```python
from build123d import *

# Parameters (mm, degrees)
SKETCH2_R           = 125
BOSS_EXTRUDE1_DEPTH = 50
CUT_EXTRUDE1_START  = -30
CUT_EXTRUDE1_DEPTH  = 30


with BuildPart() as part:
    # Sketch2 → Boss-Extrude1 (new body)
    with BuildSketch(Plane(origin=(0, 0, 0), x_dir=(1, 0, 0), z_dir=(0, 1, 0))):
        with Locations(Location((0, 0, 0), (0, 0, 270))):
            Circle(SKETCH2_R)
    extrude(amount=BOSS_EXTRUDE1_DEPTH)

    # Sketch3 → Cut-Extrude1 (cut)
    with BuildSketch(Plane(origin=(0, 50, 0), x_dir=(1, 0, 0), z_dir=(0, 1, 0)).offset(CUT_EXTRUDE1_START)):
        with BuildLine():
            Line((-122.662612071, 24.06), (122.662612071, 24.06))
            ThreePointArc((122.662612071, 24.06), (111.692828355, 56.122295874), (92.51441185, 84.06))
            Line((92.51441185, 84.06), (-92.51441185, 84.06))
            ThreePointArc((-92.51441185, 84.06), (-111.692828355, 56.122295874), (-122.662612071, 24.06))
        make_face()
        with BuildLine():
            Line((-122.662612071, -24.06), (122.662612071, -24.06))
            ThreePointArc((122.662612071, -24.06), (111.692828355, -56.122295874), (92.51441185, -84.06))
            Line((92.51441185, -84.06), (-92.51441185, -84.06))
            ThreePointArc((-92.51441185, -84.06), (-111.692828355, -56.122295874), (-122.662612071, -24.06))
        make_face()
    extrude(amount=CUT_EXTRUDE1_DEPTH, mode=Mode.SUBTRACT)


solid = part.part
```
Here's how the part is built. I have some questions about the finished solid (model axes, mm). A direction names the side the tool comes from. Coordinates: 2 decimals unless noted, no trailing zeros. Write each loop counter-clockwise with the first axis right and the second up, starting at its lowest first coordinate (ties: lowest second). Pieces come first, ordered by that corner, then holes. Notation, with made-up numbers: (46.5, -12) -> (103.5, -12) arc R20 ccw to (103.5, 17) -> close; hole circle Ø5 at (-8, 77.25). An arc over 180 degrees is marked (long way). Use a Markdown table: item, result. Add a question column.
(1) If we section it at B-B, the plane x = 0: Write out the boundary of the cut face in (y, z), and give its area (3 significant figures).
(2) If we section it at C-C, the plane z = -35: Write out the boundary of the cut face in (x, y), and give its area (3 significant figures).
(3) I'm going to push flat-ended pins straight in: P1, Ø6, axis at x = 84, z = -77.5, coming from the +Y side; P2, Ø1.5, axis at y = 44, z = -94, coming from the -X side; P3, Ø3, axis at y = 24, z = 26.5, coming from the -X side; P4, Ø9, axis at x = 23, y = 37, coming from the -Z side. Where does each tip first touch, or does it pass through?
(4) If we section it at A-A, the plane y = 41: Write out the boundary of the cut face in (x, z).
(5) We'd pull the mould along Z, two halves only. Please class faces 3 (the cylindrical face through (84.48, 24.65, -92.13)), 4 (the flat face through (2, 0, -2)), 5 (the flat face through (-2, 35, 24.06)): +Z half, -Z half, draft (parallel to the pull), parting line (faces both ways), or undercut.
(6) For faces 1 (the flat face through (1, 35, 84.06)), 2 (the flat face through (1, 50, 100)), which set-ups out of +Z, -Z, +X, -X, +Y, -Y let a thin tool reach every point of the face, with its end or its side?
(7) Please list where these lines run through material, in increasing order: line 1 (Z direction, x = -84, y = 39); line 2 (Z direction, x = -22, y = 26); line 3 (Z direction, x = -101.5, y = 20.5).
(8) If we section it at D-D, the plane y = 16: Write out the boundary of the cut face in (x, z), and give its area (3 significant figures).
Outcome:
| question | item | result |
|---|---|---|
| 1 | outline | (0, -125) -> (50, -125) -> (50, -84.06) -> (20, -84.06) -> (20, -24.06) -> (50, -24.06) -> (50, 24.06) -> (20, 24.06) -> (20, 84.06) -> (50, 84.06) -> (50, 125) -> (0, 125) -> close |
| 1 | area | 8,900 mm^2 |
| 2 | outline | (-120, 0) -> (120, 0) -> (120, 20) -> (-120, 20) -> close |
| 2 | area | 4,800 mm^2 |
| 3 | P1 | stops at y = 20 |
| 3 | P2 | stops at x = -83.24 |
| 3 | P3 | passes through |
| 3 | P4 | stops at z = -123.62 |
| 4 | outline | (-122.66, -24.06) -> (122.66, -24.06) arc R125 ccw to (122.66, 24.06) -> (-122.66, 24.06) arc R125 ccw to start; (-92.51, -84.06) arc R125 ccw to (92.51, -84.06) -> close; (-92.51, 84.06) -> (92.51, 84.06) arc R125 ccw to start |
| 5 | face 3 | parting line |
| 5 | face 4 | draft |
| 5 | face 5 | undercut |
| 6 | face 1 | +X, -X, +Y |
| 6 | face 2 | +Z, -Z, +X, -X, +Y |
| 7 | line 1 | z = -92.57 to -84.06, -24.06 to 24.06, 84.06 to 92.57 |
| 7 | line 2 | z = -123.05 to -84.06, -24.06 to 24.06, 84.06 to 123.05 |
| 7 | line 3 | z = -24.06 to 24.06 |
| 8 | outline | circle Ø250 at (0, 0) |
| 8 | area | 49,100 mm^2 |
